Autodesk Inventor part; units mm, degrees
ref_plane "2p1_XY" through (0, 0, 0) normal (0, 0, -1) x (1, 0, 0)
ref_plane "2p1_YZ" through (0, 0, 0) normal (1, 0, 0) x (0, -1, 0)
ref_plane "2p1_ZX" through (0, 0, 0) normal (0, -1, 0) x (0, 0, -1)
sketch "Sketch_1" plane through (0, 0, 0) normal (1, 0, 0) x (0, 1, 0)
  line L0 (-18.5, 0) -> (-18.5, -17.6)
  line L1 (-18.5, -17.6) -> (-14, -23.1)
  line L2 (-14, -23.1) -> (14, -23.1)
  line L3 (14, -23.1) -> (18.5, -17.6)
  line L4 (18.5, -17.6) -> (18.5, 0)
  line L5 (18.5, 0) -> (-18.5, 0)
extrude "Extrusion1" add sketch "Sketch_1" along normal blind 20
sketch "Sketch_2" plane through (0, 0, 0) normal (0, 0, 1) x (1, 0, 0)
  line L0 (0, 18.5) -> (20, 18.5)
  line L1 (20, 18.5) -> (18.15, 19.3)
  line L2 (18.15, 19.3) -> (1.85, 19.3)
  line L3 (1.85, 19.3) -> (0, 18.5)
extrude "Extrusion2" add sketch "Sketch_2" against normal blind 15.1
sketch "Sketch_3" plane through (0, 0, 0) normal (0, 0, 1) x (1, 0, 0)
  line L0 (0, -18.5) -> (1.85, -19.3)
  line L1 (1.85, -19.3) -> (18.15, -19.3)
  line L2 (18.15, -19.3) -> (20, -18.5)
  line L3 (20, -18.5) -> (0, -18.5)
extrude "Extrusion3" add sketch "Sketch_3" against normal blind 15.1
sketch "Sketch_4" plane through (0, 0, 0) normal (0, 0, 1) x (1, 0, 0)
  line L0 (-0.5, 18.272) -> (-0.5, 14.3)
  line L1 (-0.5, 14.3) -> (0.5, 14.3)
  line L2 (0.5, 14.3) -> (0.5, 18.7044)
  line L3 (0.5, 18.7044) -> (-0.5, 18.272)
extrude "Extrusion4" add sketch "Sketch_4" against normal blind 4
sketch "Sketch_5" plane through (0, 0, 0) normal (0, 0, 1) x (1, 0, 0)
  line L0 (19.5, 18.7044) -> (19.5, 14.3)
  line L1 (19.5, 14.3) -> (20.1, 14.3)
  arc A0 (20.1, 14.3) -> (20.5, 14.7) centre (20.1, 14.7) ccw
  line L2 (20.5, 14.7) -> (20.5, 18.272)
  line L3 (20.5, 18.272) -> (19.5, 18.7044)
extrude "Extrusion5" add sketch "Sketch_5" against normal blind 4
sketch "Sketch_6" plane through (0, 0, 0) normal (0, 0, 1) x (1, 0, 0)
  line L0 (-0.5, -18.272) -> (0.5, -18.7044)
  line L1 (0.5, -18.7044) -> (0.5, -14.3)
  line L2 (0.5, -14.3) -> (-0.5, -14.3)
  line L3 (-0.5, -14.3) -> (-0.5, -18.272)
extrude "Extrusion6" add sketch "Sketch_6" against normal blind 4
sketch "Sketch_7" plane through (0, 0, 0) normal (0, 0, 1) x (1, 0, 0)
  line L0 (19.5, -18.7044) -> (20.5, -18.272)
  line L1 (20.5, -18.272) -> (20.5, -14.7)
  arc A0 (20.5, -14.7) -> (20.1, -14.3) centre (20.1, -14.7) ccw
  line L2 (20.1, -14.3) -> (19.5, -14.3)
  line L3 (19.5, -14.3) -> (19.5, -18.7044)
extrude "Extrusion7" add sketch "Sketch_7" against normal blind 4
sketch "Sketch_8" plane through (20, 0, 0) normal (1, 0, 0) x (0, 0, -1)
  circle A0 centre (16.3, 16.5) radius 1.5
extrude "Extrusion8" add sketch "Sketch_8" along normal mid plane 2
sketch "Sketch_9" plane through (20, 0, 0) normal (1, 0, 0) x (0, 0, -1)
  circle A0 centre (16.3, -16.5) radius 1.5
extrude "Extrusion9" add sketch "Sketch_9" along normal mid plane 2
sketch "Sketch_10" plane through (5.55, 0, 0) normal (1, 0, 0) x (0, 0, -1)
  line L0 (0.8, 8) -> (-1.2, 8)
  line L1 (-1.2, 8) -> (-1.2, 12.05)
  line L2 (-1.2, 12.05) -> (0, 12.05)
  arc A0 (0, 12.05) -> (0.8, 11.25) centre (0.8, 12.05) ccw
  line L3 (0.8, 11.25) -> (0.8, 8)
  line L4 (0.8, 8) -> (-1.2, 8)
revolve "Revolution1" cut sketch "Sketch_10" angle 360 about axis through (5.55, 8, -0.8) along (0, 0, -1)
sketch "Sketch_11" plane through (14.45, 0, 0) normal (1, 0, 0) x (0, 0, -1)
  line L0 (0.8, 8) -> (-1.2, 8)
  line L1 (-1.2, 8) -> (-1.2, 12.05)
  line L2 (-1.2, 12.05) -> (0, 12.05)
  arc A0 (0, 12.05) -> (0.8, 11.25) centre (0.8, 12.05) ccw
  line L3 (0.8, 11.25) -> (0.8, 8)
  line L4 (0.8, 8) -> (-1.2, 8)
revolve "Revolution2" cut sketch "Sketch_11" angle 360 about axis through (14.45, 8, -0.8) along (0, 0, -1)
sketch "Sketch_12" plane through (5.55, 0, 0) normal (1, 0, 0) x (0, 0, -1)
  line L0 (0.8, -8) -> (-1.2, -8)
  line L1 (-1.2, -8) -> (-1.2, -3.95)
  line L2 (-1.2, -3.95) -> (0, -3.95)
  arc A0 (0, -3.95) -> (0.8, -4.75) centre (0.8, -3.95) ccw
  line L3 (0.8, -4.75) -> (0.8, -8)
  line L4 (0.8, -8) -> (-1.2, -8)
revolve "Revolution3" cut sketch "Sketch_12" angle 360 about axis through (5.55, -8, -0.8) along (0, 0, -1)
sketch "Sketch_13" plane through (14.45, 0, 0) normal (1, 0, 0) x (0, 0, -1)
  line L0 (0.8, -8) -> (-1.2, -8)
  line L1 (-1.2, -8) -> (-1.2, -3.95)
  line L2 (-1.2, -3.95) -> (0, -3.95)
  arc A0 (0, -3.95) -> (0.8, -4.75) centre (0.8, -3.95) ccw
  line L3 (0.8, -4.75) -> (0.8, -8)
  line L4 (0.8, -8) -> (-1.2, -8)
revolve "Revolution4" cut sketch "Sketch_13" angle 360 about axis through (14.45, -8, -0.8) along (0, 0, -1)
sketch "Sketch_14" plane through (20, 0, 0) normal (1, 0, 0) x (0, 0, -1)
  line L0 (2.9, 5.6) -> (2.9, 3.75)
  line L1 (2.9, 3.75) -> (7.8, 3.75)
  arc A0 (7.8, 3.75) -> (8.3, 4.25) centre (7.8, 4.25) ccw
  line L2 (8.3, 4.25) -> (8.3, 5.1)
  arc A1 (8.3, 5.1) -> (7.8, 5.6) centre (7.8, 5.1) ccw
  line L3 (7.8, 5.6) -> (2.9, 5.6)
extrude "Extrusion10" add sketch "Sketch_14" along normal mid plane 7.8
sketch "Sketch_15" plane through (20, 0, 0) normal (1, 0, 0) x (0, 0, -1)
  line L0 (2.9, -3.75) -> (2.9, -5.6)
  line L1 (2.9, -5.6) -> (7.8, -5.6)
  arc A0 (7.8, -5.6) -> (8.3, -5.1) centre (7.8, -5.1) ccw
  line L2 (8.3, -5.1) -> (8.3, -4.25)
  arc A1 (8.3, -4.25) -> (7.8, -3.75) centre (7.8, -4.25) ccw
  line L3 (7.8, -3.75) -> (2.9, -3.75)
extrude "Extrusion11" add sketch "Sketch_15" along normal mid plane 7.8
sketch "Sketch_16" plane through (23.9, 0, 0) normal (1, 0, 0) x (0, 0, -1)
  line L0 (1.8, 3.75) -> (8.0083, 3.75)
  line L1 (8.0083, 3.75) -> (7.5053, 8)
  line L2 (7.5053, 8) -> (1.8, 8)
  line L3 (1.8, 8) -> (1.8, 3.75)
extrude "Extrusion12" add sketch "Sketch_16" against normal blind 1.3
sketch "Sketch_17" plane through (23.9, 0, 0) normal (1, 0, 0) x (0, 0, -1)
  line L0 (1.8, -3.75) -> (1.8, -8)
  line L1 (1.8, -8) -> (7.5053, -8)
  line L2 (7.5053, -8) -> (8.0083, -3.75)
  line L3 (8.0083, -3.75) -> (1.8, -3.75)
extrude "Extrusion13" add sketch "Sketch_17" against normal blind 1.3
sketch "Sketch_19" plane through (20, 0, 0) normal (1, 0, 0) x (0, 0, -1)
  line L0 (4, 3.75) -> (4, 0.75)
  line L1 (4, 0.75) -> (7.4, 0.75)
  arc A0 (7.4, 0.75) -> (8.4, 1.75) centre (7.4, 1.75) ccw
  line L2 (8.4, 1.75) -> (8.4, 2.75)
  arc A1 (8.4, 2.75) -> (7.4, 3.75) centre (7.4, 2.75) ccw
  line L3 (7.4, 3.75) -> (4, 3.75)
extrude "Extrusion14" cut sketch "Sketch_19" along normal mid plane 1.1
sketch "Sketch_20" plane through (20, 0, 0) normal (1, 0, 0) x (0, 0, -1)
  line L0 (4, -0.75) -> (4, -3.75)
  line L1 (4, -3.75) -> (7.4, -3.75)
  arc A0 (7.4, -3.75) -> (8.4, -2.75) centre (7.4, -2.75) ccw
  line L2 (8.4, -2.75) -> (8.4, -1.75)
  arc A1 (8.4, -1.75) -> (7.4, -0.75) centre (7.4, -1.75) ccw
  line L3 (7.4, -0.75) -> (4, -0.75)
extrude "Extrusion15" cut sketch "Sketch_20" along normal mid plane 1.1
sketch "Sketch_21" plane through (20, 0, 0) normal (1, 0, 0) x (0, 0, -1)
  circle A0 centre (5.65, 2.25) radius 0.8
extrude "Extrusion16" add sketch "Sketch_21" along normal mid plane 20
sketch "Sketch_22" plane through (20, 0, 0) normal (1, 0, 0) x (0, 0, -1)
  circle A0 centre (5.65, -2.25) radius 0.8
extrude "Extrusion17" add sketch "Sketch_22" along normal mid plane 20
ref_plane "2p1_XY" through (0, 0, 0) normal (0, 0, -1) x (1, 0, 0)
ref_plane "2p1_YZ" through (0, 0, 0) normal (1, 0, 0) x (0, -1, 0)
ref_plane "2p1_ZX" through (0, 0, 0) normal (0, -1, 0) x (0, 0, -1)
properties part number "259434_part2"
The model under review builds one solid part; all positions refer to its coordinate system, in mm. A direction names the side the tool comes from. Round coordinates to 2 decimals unless told otherwise and drop trailing zeros. Loops run counter-clockwise (first coordinate to the right, second up) from the corner with the lowest first, then second, coordinate; pieces in that order, holes last. Notation, with made-up numbers: (-30.5, 58.5) - (-23.5, 58.5) arc R15 ccw to (-23.5, 64.5) - close; hole circle Ø6 at (78, -33.5). An arc over 180 degrees is marked (long way). Use a Markdown table: item, result. Add a question column.
Q1. The part is to be moulded in two halves that separate along X. For faces 1 (the face through (19.45, -2, -7)), 2 (the face through (22.6, 6, -4)), 3 (the face through (19.721, 1.051, -8.115)), say which applies: pulls with the +X half, pulls with the -X half, needs draft (parallel to the pull), parting line crosses it, or undercut.
Q2. Machinability: for faces 4 (the face through (19.721, 3.465, -8.099)), 5 (the face through (23.259, -6.817, -7.645)), 6 (the face through (20.5, -17, -2)), 7 (the face through (22.6, -6, -4)), 8 (the face through (10, -18.5, -16)), which of the approach directions +Z, -Z, +X, -X, +Y, -Y give a long, thin tool a straight path to every point of the face, cutting with its end or side? Answer none if there is none.
Q3. Add section C-C (z = -16.3). State the section outline as (x, y) points.
Q4. Add section A-A (x = 22). State the section outline as (y, z) points.
Q5. Insertion check: pin 1 Ø8 at (y, z) = (15.5, -17.5) entering from -X; pin 2 Ø5 at (x, y) = (4.5, -7) entering from +Z; pin 3 Ø0.6 at (x, y) = (21, 4.5) entering from +Z. Each pin has a flat end and moves straight along its axis. Give the tip position at first contact, or say it passes through.
Q6. For probe 1 along Y at (x, z) = (20.5, -5.75); probe 2 along X at (y, z) = (-12.5, -21.75); probe 3 along Y at (x, z) = (25, -5.5), list the stretches that pass through material, from the lowest coordinate up.
Q7. Add section D-D (x = 27). State the section outline as (y, z) points.
Q8. Add section B-B (y = 2.25). State the section outline as (x, z) points, plus the area to 3 significant figures.
Worked answers:
| question | item | result |
|---|---|---|
| 1 | face 1 | pulls with the +X half |
| 1 | face 2 | undercut |
| 1 | face 3 | needs draft |
| 2 | face 4 | +X |
| 2 | face 5 | -Z, +X, -Y |
| 2 | face 6 | +Z, +X, -Y |
| 2 | face 7 | +Z, -Y |
| 2 | face 8 | -Z, +X, -X, -Y |
| 3 | outline | (0, -18.5) - (20, -18.5) - (20, -18) - (21, -18) - (21, -15) - (20, -15) - (20, 15) - (21, 15) - (21, 18) - (20, 18) - (20, 18.5) - (0, 18.5) - close |
| 4 | outline | (-5.6, -7.8) arc R0.5 ccw to (-5.1, -8.3) - (-4.25, -8.3) arc R0.5 ccw to (-3.75, -7.8) - (-3.75, -2.9) - (-5.6, -2.9) - close; circle Ø1.6 at (-2.25, -5.65); circle Ø1.6 at (2.25, -5.65); (3.75, -7.8) arc R0.5 ccw to (4.25, -8.3) - (5.1, -8.3) arc R0.5 ccw to (5.6, -7.8) - (5.6, -2.9) - (3.75, -2.9) - close |
| 5 | pin 1 | x = 0 |
| 5 | pin 2 | z = -0.01 |
| 5 | pin 3 | z = -2.9 |
| 6 | probe 1 | -5.6 to -3.75, -3.04 to -1.46, 1.46 to 3.04, 3.75 to 5.6 |
| 6 | probe 2 | 0 to 20 |
| 6 | probe 3 | -3.04 to -1.46, 1.46 to 3.04 |
| 7 | outline | circle Ø1.6 at (-2.25, -5.65); circle Ø1.6 at (2.25, -5.65) |
| 8 | outline | (0, -23.1) - (20, -23.1) - (20, -8.4) - (19.45, -8.4) - (19.45, -6.45) - (30, -6.45) - (30, -4.85) - (19.45, -4.85) - (19.45, -4) - (20, -4) - (20, 0) - (0, 0) - close |
| 8 | area | 476 mm² |
